Build history of the part. All positions in model axes, mm. Coordinates: 2 decimals unless noted, no trailing zeros. Order: outer loops, then holes, each group sorted by start corner. A loop starts at its lowest first (then second) coordinate and runs counter-clockwise, first axis right, second up. Notation, with made-up numbers: M -15.5,83.5 L 31.5,83.5 A21 ccw 31.5,92.5 Z; hole C 27.5,-12 d2. An arc over 180 degrees is marked long. Write item = value, one per line. Start each with the question number.
Q1. Pin check, flat tips, straight feed: P1, Ø2.5, axis at x = 23, y = 5, coming from the -Z side; P2, Ø1, axis at x = 77.5, z = 2, coming from the +Y side; P3, Ø1.5, axis at y = 41.5, z = 0.5, coming from the +X side. Stop position of each tip, or through.
Q2. Drill centre lines: probe 1 along X at (y, z) = (4, 1.8); probe 2 along X at (y, z) = (5, 1); probe 3 along Y at (x, z) = (23, 0.6). Where is each one in solid material? Low to high.
Q3. Band-saw the part on B-B on z = 0.95. Write the cut outline in (x, y), plus the area to 3 significant figures.
```python
from build123d import *

# Parameters (mm, degrees)
SKETCH1_W                                      = 193
SKETCH1_H                                      = 54
BOSS_EXTRUDE1_DEPTH                            = 3
CHAMFER1_SIZE                                  = 3
CSK_FOR_M3_FLAT_HEAD_MACHINE_SCREW1_AT_2_COUNT = 2
CSK_FOR_M3_FLAT_HEAD_MACHINE_SCREW1_AT_2_PITCH = 73.5
CSK_FOR_M3_FLAT_HEAD_MACHINE_SCREW1_AT_3_COUNT = 2
CSK_FOR_M3_FLAT_HEAD_MACHINE_SCREW1_AT_3_PITCH = 147


with BuildPart() as part:
    # Sketch1 → Boss-Extrude1 (new body)
    with BuildSketch(Plane.XY):
        with Locations((96.5, 27)):
            Rectangle(SKETCH1_W, SKETCH1_H)
    extrude(amount=BOSS_EXTRUDE1_DEPTH)

    # Chamfer1
    chamfer1_edges = [part.edges().sort_by_distance(p)[0] for p in [
        (0, 27, 0),
        (96.5, 54, 0),
        (193, 27, 0),
    ]]
    chamfer(chamfer1_edges, length=CHAMFER1_SIZE - 0.0001)  # a hair under: the kernel refuses the full size

    # Sketch3 → CSK for M3 Flat Head Machine Screw1 (revolve, cut)
    with BuildSketch(Plane(origin=(23, 5, 3), x_dir=(0, -1, 0), z_dir=(1, 0, 0))):
        Polygon((0, 0), (0, 3), (1.7, 3), (1.7, 1.45), (3.15, 0), align=None)
    csk_for_m3_flat_head_machine_screw1 = revolve(axis=Axis((23, 5, 9.35), (0, 0, -1)), mode=Mode.SUBTRACT)

    # CSK for M3 Flat Head Machine Screw1 at 2: CSK for M3 Flat Head Machine Screw1 ×2
    with Locations(*[(i * CSK_FOR_M3_FLAT_HEAD_MACHINE_SCREW1_AT_2_PITCH, 0, 0) for i in range(1, CSK_FOR_M3_FLAT_HEAD_MACHINE_SCREW1_AT_2_COUNT)]):
        add(csk_for_m3_flat_head_machine_screw1, mode=Mode.SUBTRACT)

    # CSK for M3 Flat Head Machine Screw1 at 3: CSK for M3 Flat Head Machine Screw1 ×2
    with Locations(*[(i * CSK_FOR_M3_FLAT_HEAD_MACHINE_SCREW1_AT_3_PITCH, 0, 0) for i in range(1, CSK_FOR_M3_FLAT_HEAD_MACHINE_SCREW1_AT_3_COUNT)]):
        add(csk_for_m3_flat_head_machine_screw1, mode=Mode.SUBTRACT)


solid = part.part
```
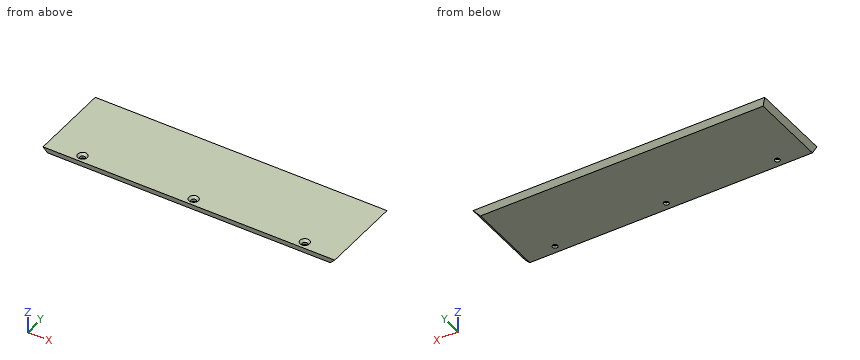
Recorded:
q1.P1 = through
q1.P2 = 53.5
q1.P3 = 191.25
q2.probe_1 = 1.2 to 21.33, 24.67 to 94.83, 98.17 to 168.33, 171.67 to 191.8
q2.probe_2 = 2 to 21.3, 24.7 to 94.8, 98.2 to 168.3, 171.7 to 191
q2.probe_3 = 0 to 3.3, 6.7 to 51.6
q3.outline = M 2.05,0 L 190.95,0 L 190.95,51.95 L 2.05,51.95 Z; hole C 23,5 d3.4; hole C 96.5,5 d3.4; hole C 170,5 d3.4
q3.area = 9,790 mm2
